Read the model definition and answer for the solid it produces. Units are mm, in the model's axes. Coordinates: 2 decimals unless noted, no trailing zeros. Loops run counter-clockwise (first coordinate to the right, second up) from the corner with the lowest first, then second, coordinate; pieces in that order, holes last. Notation, with made-up numbers: (9.25, 65) -> (57.25, 65) arc R8 cw to (57.25, 69) -> close; hole circle Ø4 at (74.25, 7). An arc over 180 degrees is marked (long way). Answer as a JSON object with one key per item and string values. Group by question number.
Q1. The part is cut by section A-A on z = 21. Write down the section's boundary in (x, y) (1 decimal), and give its area (3 significant figures).
Q2. Each of these flat-tipped pins is pushed along its axis until it touches: P1, Ø1, axis at x = -4, y = 1, coming from the -Z side; P2, Ø1.8, axis at x = -0.5, y = 1, coming from the -Z side. Where does it stop, or does it pass through?
Q3. Straight lines are drawn through the part: line 1 along X through (y, z) = (-3.75, 119); line 2 along Z through (x, y) = (-0.25, -1) (3 decimals); line 3 along X through (y, z) = (2.25, 133.5). For each, find the intervals that lie inside material, in ascending order. Write a range as [from, to].
from build123d import *

# Parameters (mm, degrees)
BOSS_EXTRUDE1_DEPTH = 179.705
CUT_EXTRUDE1_DEPTH  = 6.35
CUT_EXTRUDE2_DEPTH  = 6.35


with BuildPart() as part:
    # Sketch1 → Boss-Extrude1 (new body)
    with BuildSketch(Plane.XY):
        Polygon((5.715, 0), (2.8575, 4.949335183), (-2.8575, 4.949335183), (-5.715, 0), (-2.8575, -4.949335183), (2.8575, -4.949335183), align=None)
    extrude(amount=BOSS_EXTRUDE1_DEPTH)

    # Sketch2 → Cut-Extrude1 (cut)
    with BuildSketch(Plane.XY.offset(179.705)):
        Polygon((3.521836637, 0), (1.760918319, 3.049999996), (-1.760918319, 3.049999996), (-3.521836637, 0), (-1.760918319, -3.049999996), (1.760918319, -3.049999996), align=None)
    extrude(amount=-CUT_EXTRUDE1_DEPTH, mode=Mode.SUBTRACT)

    # Sketch3 → Cut-Extrude2 (cut)
    with BuildSketch(Plane(origin=(0, 0, 0), x_dir=(-1, 0, 0), z_dir=(0, 0, -1))):
        Polygon((1.760918319, 3.049999996), (-1.760918319, 3.049999996), (-3.521836637, 0), (-1.760918319, -3.049999996), (1.760918319, -3.049999996), (3.521836637, 0), align=None)
    extrude(amount=-CUT_EXTRUDE2_DEPTH, mode=Mode.SUBTRACT)


solid = part.part
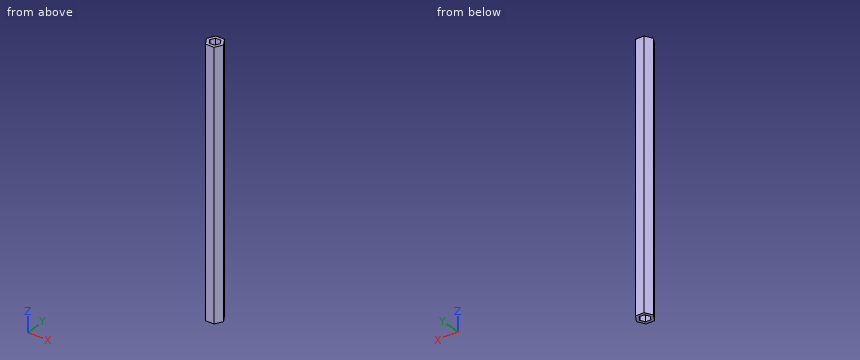
Final values:
{
 "1": {"outline": "(-5.7, 0) -> (-2.9, -4.9) -> (2.9, -4.9) -> (5.7, 0) -> (2.9, 4.9) -> (-2.9, 4.9) -> close", "area": "84.9 mm2"},
 "2": {"P1": "stops at z = 0", "P2": "stops at z = 6.35"},
 "3": {"line 1": "x = [-3.55, 3.55]", "line 2": "z = [6.35, 173.355]", "line 3": "x = [-4.42, 4.42]"}
}
